Source: CAD feature listing. Evaluate the final solid. Frame: model axes, mm. Face numbers are marked on the shaded views. A direction names the side the tool comes from. Coordinates: 2 decimals unless noted, no trailing zeros. Write each loop counter-clockwise with the first axis right and the second up, starting at its lowest first coordinate (ties: lowest second). Pieces come first, ordered by that corner, then holes. Notation, with made-up numbers: (10, 51.5) - (40, 51.5) arc R6 cw to (40, 60.5) - close; hole circle Ø1 at (74.25, 42.5). An arc over 180 degrees is marked (long way). One line per item, written item: value.
from build123d import *
from build123d import SkipClean  # not in build123d's __all__

# Parameters (mm, degrees)
F0_R      = 3
F0_R_2    = 1.8
F1_DEPTH  = 13
F2_R      = 1.8
F3_DEPTH  = 1.5
F4_W      = 6
F4_H      = 6
F5_DEPTH  = 1
F6_W      = 15.15
F6_H      = 11.5
F7_DEPTH  = 5.8
F8_W      = 12.75
F8_H      = 7
F9_DEPTH  = 4.6
F10_W     = 11.75
F10_H     = 3.56
F11_DEPTH = 4
F13_DEPTH = 2
F15_DEPTH = 25


with BuildPart() as f1:
    # F0 (on Top) → F1 (new body)
    with BuildSketch(Plane.XY):
        with Locations((-14, 14)):
            Circle(F0_R)
        with Locations((-14, 14)):
            Circle(F0_R_2, mode=Mode.SUBTRACT)
    extrude(amount=F1_DEPTH)



with BuildPart() as f1b:
    # F0 (on Top) → F1, piece 2 (new body)
    with BuildSketch(Plane.XY):
        with Locations((-14, -14)):
            Circle(F0_R)
        with Locations((-14, -14)):
            Circle(F0_R_2, mode=Mode.SUBTRACT)
    extrude(amount=F1_DEPTH)


with BuildPart() as f1c:
    # F0 (on Top) → F1, piece 3 (new body)
    with BuildSketch(Plane.XY):
        with Locations((14, -14)):
            Circle(F0_R)
        with Locations((14, -14)):
            Circle(F0_R_2, mode=Mode.SUBTRACT)
    extrude(amount=F1_DEPTH)


with BuildPart() as f1d:
    # F0 (on Top) → F1, piece 4 (new body)
    with BuildSketch(Plane.XY):
        with Locations((14, 14)):
            Circle(F0_R)
        with Locations((14, 14)):
            Circle(F0_R_2, mode=Mode.SUBTRACT)
    extrude(amount=F1_DEPTH)


with BuildPart() as f1_1:
    add(f1.part, clean=False)

    with SkipClean():  # cleaning this boolean's faces spoils the solid; the shape is the same uncleaned
        add(f1b.part)  # F3 merges F1b

    with SkipClean():  # cleaning this boolean's faces spoils the solid; the shape is the same uncleaned
        add(f1c.part)  # F3 merges F1c

    with SkipClean():  # cleaning this boolean's faces spoils the solid; the shape is the same uncleaned
        add(f1d.part)  # F3 merges F1d
    # F2 (on face) → F3 (join)
    with BuildSketch(Plane.XY.offset(13)):
        with BuildLine():
            Line((14, 17), (-14, 17))
            ThreePointArc((-14, 17), (-16.1213203436, 16.1213203436), (-17, 14))
            Line((-17, 14), (-17, -14))
            ThreePointArc((-17, -14), (-16.1213203436, -16.1213203436), (-14, -17))
            Line((-14, -17), (14, -17))
            ThreePointArc((14, -17), (16.1213203436, -16.1213203436), (17, -14))
            Line((17, -14), (17, 14))
            ThreePointArc((17, 14), (16.1213203436, 16.1213203436), (14, 17))
        make_face()
        with Locations((-14, -14)):
            Circle(F2_R, mode=Mode.SUBTRACT)
        with Locations((14, -14)):
            Circle(F2_R, mode=Mode.SUBTRACT)
        with Locations((-14, 14)):
            Circle(F2_R, mode=Mode.SUBTRACT)
        with BuildLine():
            Line((-15, -11.1715728753), (-15, 11.1715728753))
            ThreePointArc((-15, 11.1715728753), (-11.8786796564, 11.8786796564), (-11.1715728753, 15))
            Line((-11.1715728753, 15), (11.1715728753, 15))
            ThreePointArc((11.1715728753, 15), (11.8786796564, 11.8786796564), (15, 11.1715728753))
            Line((15, 11.1715728753), (15, -11.1715728753))
            ThreePointArc((15, -11.1715728753), (11.8786796564, -11.8786796564), (11.1715728753, -15))
            Line((11.1715728753, -15), (-11.1715728753, -15))
            ThreePointArc((-11.1715728753, -15), (-11.8786796564, -11.8786796564), (-15, -11.1715728753))
        make_face(mode=Mode.SUBTRACT)
        with Locations((14, 14)):
            Circle(F2_R, mode=Mode.SUBTRACT)
    with SkipClean():  # cleaning this boolean's faces spoils the solid; the shape is the same uncleaned
        extrude(amount=F3_DEPTH)

    # F4 (on face) → F5 (join)
    with BuildSketch(Plane.XY.offset(14.5)):
        Polygon((1, 15), (-1, 15), (-1, 9), (-7, 9), (-7, 15), (-9, 15), (-9, 9), (-15, 9), (-15, 7), (-9, 7), (-9, 1), (-15, 1), (-15, -1), (-9, -1), (-9, -7), (-15, -7), (-15, -9), (-9, -9), (-9, -15), (-7, -15), (-7, -9), (-1, -9), (-1, -15), (1, -15), (1, -9), (7, -9), (7, -15), (9, -15), (9, -9), (15, -9), (15, -7), (9, -7), (9, -1), (15, -1), (15, 1), (9, 1), (9, 7), (15, 7), (15, 9), (9, 9), (9, 15), (7, 15), (7, 9), (1, 9), align=None)
        with Locations((-4, -4)):
            Rectangle(F4_W, F4_H, mode=Mode.SUBTRACT)
        with Locations((4, -4)):
            Rectangle(F4_W, F4_H, mode=Mode.SUBTRACT)
        with Locations((-4, 4)):
            Rectangle(F4_W, F4_H, mode=Mode.SUBTRACT)
        with Locations((4, 4)):
            Rectangle(F4_W, F4_H, mode=Mode.SUBTRACT)
    extrude(amount=-F5_DEPTH)

    # F6 (on face) → F7 (join)
    with BuildSketch(Plane.XY.offset(14.5)):
        with Locations((0, 22.75)):
            Rectangle(F6_W, F6_H)
    with SkipClean():  # cleaning this boolean's faces spoils the solid; the shape is the same uncleaned
        extrude(amount=-F7_DEPTH)

    # F8 (on face) → F9 (cut)
    with BuildSketch(Plane(origin=(0, 0, 8.7), x_dir=(1, 0, 0), z_dir=(0, 0, -1))):
        with Locations((0, -20.5)):
            Rectangle(F8_W, F8_H)
    with SkipClean():  # cleaning this boolean's faces spoils the solid; the shape is the same uncleaned
        extrude(amount=-F9_DEPTH, mode=Mode.SUBTRACT)

    # F10 (on face) → F11 (cut)
    with BuildSketch(Plane(origin=(0, 0, 8.7), x_dir=(1, 0, 0), z_dir=(0, 0, -1))):
        with Locations((0, -25.78)):
            Rectangle(F10_W, F10_H)
    with SkipClean():  # cleaning this boolean's faces spoils the solid; the shape is the same uncleaned
        extrude(amount=-F11_DEPTH, mode=Mode.SUBTRACT)

    # F12 (on face) → F13 (cut, symmetric)
    with BuildSketch(Plane(origin=(0, 28.5, 0), x_dir=(-1, 0, 0), z_dir=(0, 1, 0))):
        with BuildLine():
            Line((-4, 8.7), (4, 8.7))
            ThreePointArc((4, 8.7), (0, 12.7), (-4, 8.7))
        make_face()
    with SkipClean():  # cleaning this boolean's faces spoils the solid; the shape is the same uncleaned
        extrude(amount=F13_DEPTH, both=True, mode=Mode.SUBTRACT)

    # F14 (on face) → F15 (cut)
    with BuildSketch(Plane(origin=(-7.575, 0, 0), x_dir=(0, -1, 0), z_dir=(-1, 0, 0))):
        Polygon((-17, 12.2429373081), (-28.5, 8.7), (-17, 8.7), align=None)
    extrude(amount=-F15_DEPTH, mode=Mode.SUBTRACT)


solid = f1_1.part
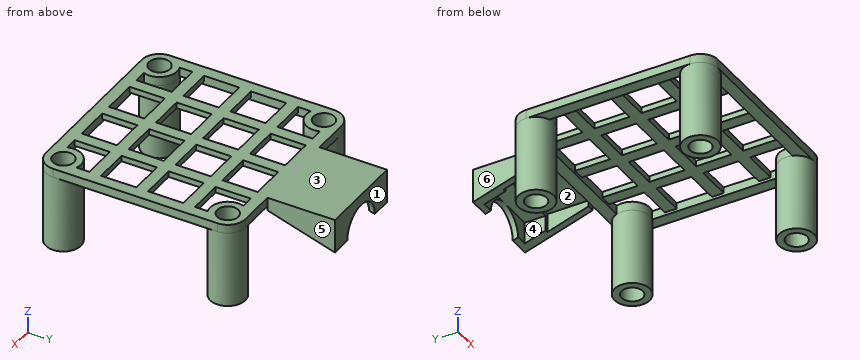
1) Section query A-A on y = 2. Output: boundary loops of the cut face in (x, z).
Values found:
outline: (-17, 13) - (-15, 13) - (-15, 14.5) - (-17, 14.5) - close; (-9, 13.5) - (-7, 13.5) - (-7, 14.5) - (-9, 14.5) - close; (-1, 13.5) - (1, 13.5) - (1, 14.5) - (-1, 14.5) - close; (7, 13.5) - (9, 13.5) - (9, 14.5) - (7, 14.5) - close; (15, 13) - (17, 13) - (17, 14.5) - (15, 14.5) - close
2) Section query B-B on z = 11.5. State how many separate pieces and enclosed holes the cut face has, then the cut area to 3 significant figures.
Values found:
separate pieces: 6
enclosed holes: 4
area: 104 mm2
3) Material intervals for line 1 (Y direction, x = -14, z = 10.5); line 2 (Y direction, x = -13, z = 6); line 3 (Y direction, x = 6, z = 10.75), sorted ascending.
Values found:
line 1: -17 to -15.8, -12.2 to -11, 11 to 12.2, 15.8 to 17
line 2: -16.83 to -15.5, -12.5 to -11.17, 11.17 to 12.5, 15.5 to 16.83
line 3: 24 to 28.5
4) Reachability of the marked faces 4, 5 and 6 from +Z, -Z, +X, -X, +Y, -Y: full face, straight path, thin tool, end or side. Return the list, or none.
Values found:
face 4: -Z, -Y
face 5: +Z, -Z, +X, +Y
face 6: +Z, -Z, -X, +Y
5) Section query D-D on y = 23. Output: boundary loops of the cut face in (x, z) (3 decimals).
Values found:
outline: (-7.575, 10.394) - (-6.375, 10.394) - (-6.375, 13.3) - (6.375, 13.3) - (6.375, 10.394) - (7.575, 10.394) - (7.575, 14.5) - (-7.575, 14.5) - close
6) Contact query for flat-ended pins moving along their axis: P1, Ø1.7, axis at y = 21, z = 13, coming from the -X side (3 decimals); P2, Ø1.1, axis at x = -3.5, z = 11, coming from the -Y side; P3, Ø6, axis at x = -5.5, z = 3.5, coming from the +Y side; P4, Ø12, axis at x = 3, y = 23.5, coming from the -Z side. Output: stop coordinate, or through.
Values found:
P1: x = -7.575
P2: y = 27.56
P3: through
P4: z = 8.7
7) Draft query along Y for the marked faces 1, 2 and 3. Return one class per face: released by +Y, released by -Y, zero draft, split by the parting line, or undercut.
Values found:
face 1: released by +Y
face 2: undercut
face 3: zero draft
